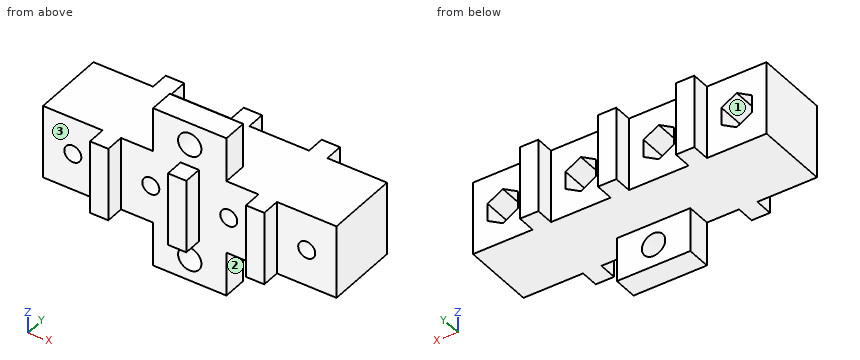
```python
from build123d import *

# Parameters (mm, degrees)
SKETCH1_W               = 50.8
SKETCH1_H               = 12.7
BOSS_EXTRUDE1_DEPTH     = 6.35
SKETCH9_W               = 3.175
SKETCH9_H               = 12.7
BOSS_EXTRUDE3_DEPTH     = 3.175
LPATTERN1_COUNT         = 3
LPATTERN1_PITCH         = 13.49375
MIRROR2_COPY_1_SKETCH_W = 3.175
MIRROR2_COPY_1_SKETCH_H = 12.7
MIRROR2_COPY_1_DEPTH    = 3.175
MIRROR2_COPY_2_SKETCH_W = 3.175
MIRROR2_COPY_2_SKETCH_H = 12.7
MIRROR2_COPY_2_DEPTH    = 3.175
CUT_EXTRUDE1_DEPTH      = 9.525
LPATTERN2_COUNT         = 4
LPATTERN2_PITCH         = 13.49375
F_4_CLEARANCE_HOLE2_D   = 2.9464
LPATTERN3_COUNT         = 4
LPATTERN3_PITCH         = 13.49375
SKETCH13_W              = 12.7
SKETCH13_H              = 4.191
BOSS_EXTRUDE4_DEPTH     = 7.62
HOLE1_D                 = 4.0386


with BuildPart() as part:
    # Sketch1 → Boss-Extrude1 (new, symmetric)
    with BuildSketch(Plane(origin=(0, 0, 0), x_dir=(1, 0, 0), z_dir=(0, 1, 0))):
        Rectangle(SKETCH1_W, SKETCH1_H)
    extrude(amount=BOSS_EXTRUDE1_DEPTH, both=True)

    # Sketch9 → Boss-Extrude3 (add)
    with BuildSketch(Plane(origin=(0, 6.35, 0), x_dir=(1, 0, 0), z_dir=(0, 1, 0))):
        with Locations((-13.49375, 0)):
            Rectangle(SKETCH9_W, SKETCH9_H)
    boss_extrude3 = extrude(amount=BOSS_EXTRUDE3_DEPTH)

    # LPattern1: Boss-Extrude3 ×3
    with Locations(*[(i * LPATTERN1_PITCH, 0, 0) for i in range(1, LPATTERN1_COUNT)]):
        add(boss_extrude3)

    # Mirror2: Boss-Extrude3 across plane
    add(boss_extrude3.mirror(Plane.ZX))

    # Mirror2 copy 1 sketch → Mirror2 copy 1 (add)
    with BuildSketch(Plane(origin=(13.49375, -6.35, 0), x_dir=(1, 0, 0), z_dir=(0, -1, 0))):
        with Locations((-13.49375, 0)):
            Rectangle(MIRROR2_COPY_1_SKETCH_W, MIRROR2_COPY_1_SKETCH_H)
    extrude(amount=MIRROR2_COPY_1_DEPTH)

    # Mirror2 copy 2 sketch → Mirror2 copy 2 (add)
    with BuildSketch(Plane(origin=(26.9875, -6.35, 0), x_dir=(1, 0, 0), z_dir=(0, -1, 0))):
        with Locations((-13.49375, 0)):
            Rectangle(MIRROR2_COPY_2_SKETCH_W, MIRROR2_COPY_2_SKETCH_H)
    extrude(amount=MIRROR2_COPY_2_DEPTH)

    # Sketch10 → Cut-Extrude1 (cut)
    with BuildSketch(Plane(origin=(0, 6.35, 0), x_dir=(1, 0, 0), z_dir=(0, 1, 0))):
        Polygon((-17.605375, 1.521462297), (-20.240625, 3.042924594), (-22.875875, 1.521462297), (-22.875875, -1.521462297), (-20.240625, -3.042924594), (-17.605375, -1.521462297), align=None)
    cut_extrude1 = extrude(amount=-CUT_EXTRUDE1_DEPTH, mode=Mode.SUBTRACT)

    # LPattern2: Cut-Extrude1 ×4
    with Locations(*[(i * LPATTERN2_PITCH, 0, 0) for i in range(1, LPATTERN2_COUNT)]):
        add(cut_extrude1, mode=Mode.SUBTRACT)

    # #4 Clearance Hole2 (through all)
    with Locations(Plane(origin=(0, -3.175, 0), x_dir=(1, 0, 0), z_dir=(0, 1, 0))):
        with Locations((-20.240625, 0)):
            f_4_clearance_hole2 = Hole(F_4_CLEARANCE_HOLE2_D / 2)

    # LPattern3: #4 Clearance Hole2 ×4
    with Locations(*[(i * LPATTERN3_PITCH, 0, 0) for i in range(1, LPATTERN3_COUNT)]):
        add(f_4_clearance_hole2, mode=Mode.SUBTRACT)

    # Sketch13 → Boss-Extrude4 (add)
    with BuildSketch(Plane.XY.offset(6.35)):
        with Locations((0, -4.2545)):
            Rectangle(SKETCH13_W, SKETCH13_H)
    boss_extrude4 = extrude(amount=BOSS_EXTRUDE4_DEPTH)

    # Hole1 (through all)
    with Locations(Plane(origin=(0, -2.159, 0), x_dir=(1, 0, 0), z_dir=(0, 1, 0))):
        with Locations((0, -10.16)):
            hole1 = Hole(HOLE1_D / 2)

    # Mirror4: Boss-Extrude4, Hole1 across plane
    add(boss_extrude4.mirror(Plane.XY))
    add(hole1.mirror(Plane.XY), mode=Mode.SUBTRACT)


solid = part.part
```
Read the model definition and answer for the solid it produces. Units are mm, in the model's axes. Face numbers are marked on the shaded views. A direction names the side the tool comes from. Give positions to 0.01 mm unless a question says otherwise; leave off trailing zeros. Write each loop counter-clockwise with the first axis right and the second up, starting at its lowest first coordinate (ties: lowest second). Pieces come first, ordered by that corner, then holes. Notation, with made-up numbers: (-34, 89.25) -> (10, 89.25) arc R22 cw to (10, 119.25) -> close; hole circle Ø5 at (-17, 7). An arc over 180 degrees is marked (long way). Answer in a Markdown table with one row per item.
1) Section C-C on z = 10.16 is taken. Give the vertices of the cut face in (x, y), plus the area to 3 significant figures.
Results list:
| item | result |
|---|---|
| outline | (-6.35, -6.35) -> (-2.02, -6.35) -> (-2.02, -2.16) -> (-6.35, -2.16) -> close; (2.02, -6.35) -> (6.35, -6.35) -> (6.35, -2.16) -> (2.02, -2.16) -> close |
| area | 36.3 mm^2 |
2) Section D-D on y = -1.5 is taken. Give the vertices of the cut face in (x, z), plus the area to 3 significant figures.
Results list:
| item | result |
|---|---|
| outline | (-25.4, -6.35) -> (25.4, -6.35) -> (25.4, 6.35) -> (-25.4, 6.35) -> close; hole (-22.88, -1.52) -> (-20.24, -3.04) -> (-17.61, -1.52) -> (-17.61, 1.52) -> (-20.24, 3.04) -> (-22.88, 1.52) -> close; hole (-9.38, -1.52) -> (-6.75, -3.04) -> (-4.11, -1.52) -> (-4.11, 1.52) -> (-6.75, 3.04) -> (-9.38, 1.52) -> close; hole (4.11, -1.52) -> (6.75, -3.04) -> (9.38, -1.52) -> (9.38, 1.52) -> (6.75, 3.04) -> (4.11, 1.52) -> close; hole (17.61, -1.52) -> (20.24, -3.04) -> (22.88, -1.52) -> (22.88, 1.52) -> (20.24, 3.04) -> (17.61, 1.52) -> close |
| area | 549 mm^2 |
3) A tool of negligible diameter and unlimited length cuts with its end or side. For the marked faces 1, 2 and 3, from which of +Z, -Z, +X, -X, +Y, -Y can it reach the whole face along a straight path? Write none if from no direction.
Results list:
| item | result |
|---|---|
| face 1 | +Y |
| face 2 | -Z, +X, +Y, -Y |
| face 3 | +Z, -Z, -X, -Y |
4) Straight lines are drawn through the part: line 1 (Z direction, x = 0, y = -3.65); line 2 (X direction, y = -6.5, z = -5); line 3 (X direction, y = -2.25, z = 11.5). For each, find the intervals that lie inside material, in ascending order. Write a range as [from, to].
Results list:
| item | result |
|---|---|
| line 1 | [-13.97, -12.18], [-8.14, 8.14], [12.18, 13.97] |
| line 2 | [-15.08, -11.91], [-1.59, 1.59], [11.91, 15.08] |
| line 3 | [-6.35, -1.51], [1.51, 6.35] |
5) Section A-A on y = -7 is taken. Give the vertices of the cut face in (x, z), plus the area to 3 significant figures.
Results list:
| item | result |
|---|---|
| outline | (-15.08, -6.35) -> (-11.91, -6.35) -> (-11.91, 6.35) -> (-15.08, 6.35) -> close; (-1.59, -6.35) -> (1.59, -6.35) -> (1.59, 6.35) -> (-1.59, 6.35) -> close; (11.91, -6.35) -> (15.08, -6.35) -> (15.08, 6.35) -> (11.91, 6.35) -> close |
| area | 121 mm^2 |
6) Section B-B on x = 0 is taken. Give the vertices of the cut face in (y, z) (3 decimals).
Results list:
| item | result |
|---|---|
| outline | (-9.525, -6.35) -> (-6.35, -6.35) -> (-6.35, -8.141) -> (-2.159, -8.141) -> (-2.159, -6.35) -> (9.525, -6.35) -> (9.525, 6.35) -> (-2.159, 6.35) -> (-2.159, 8.141) -> (-6.35, 8.141) -> (-6.35, 6.35) -> (-9.525, 6.35) -> close; (-6.35, -13.97) -> (-2.159, -13.97) -> (-2.159, -12.179) -> (-6.35, -12.179) -> close; (-6.35, 12.179) -> (-2.159, 12.179) -> (-2.159, 13.97) -> (-6.35, 13.97) -> close |
7) Each of these flat-tipped pins is pushed along its axis until it touches: pin 1 Ø3 at (x, z) = (-4.5, -0.5) entering from +Y; pin 2 Ø8 at (x, y) = (20, 5.5) entering from +Z; pin 3 Ø3.5 at (x, z) = (-20.24, 0) entering from -Y; pin 4 Ø2.5 at (x, z) = (-6.75, 0) entering from +Y. Where does it stop, or does it pass through?
Results list:
| item | result |
|---|---|
| pin 1 | y = 6.35 |
| pin 2 | z = 6.35 |
| pin 3 | y = -6.35 |
| pin 4 | through |
